```python
from build123d import *

# Parameters (mm, degrees)
SKETCH_1_W          = 20
SKETCH_1_H          = 20
SKETCH_1_W_2        = 17
SKETCH_1_H_2        = 17
EXTRUDE_1_DEPTH     = 415
SKETCH_5_R          = 1.6
CUT_EXTRUDE_4_DEPTH = 416.601973046


with BuildPart() as part:
    # 草图1 → 凸台-拉伸1 (new body)
    with BuildSketch(Plane.XY):
        Rectangle(SKETCH_1_W, SKETCH_1_H)
        Rectangle(SKETCH_1_W_2, SKETCH_1_H_2, mode=Mode.SUBTRACT)
    extrude(amount=EXTRUDE_1_DEPTH)

    # 草图5 → 切除-拉伸4 (cut, through all)
    with BuildSketch(Plane.XZ.offset(10)):
        with Locations(Location((0, 10, 0), (0, 0, 270))):
            Circle(SKETCH_5_R)
        with Locations(Location((0, 30, 0), (0, 0, 270))):
            Circle(SKETCH_5_R)
        with Locations(Location((0, 50, 0), (0, 0, 270))):
            Circle(SKETCH_5_R)
        with Locations(Location((0, 70, 0), (0, 0, 270))):
            Circle(SKETCH_5_R)
        with Locations(Location((0, 90, 0), (0, 0, 270))):
            Circle(SKETCH_5_R)
        with Locations(Location((0, 110, 0), (0, 0, 270))):
            Circle(SKETCH_5_R)
        with Locations(Location((0, 130, 0), (0, 0, 270))):
            Circle(SKETCH_5_R)
        with Locations(Location((0, 150, 0), (0, 0, 270))):
            Circle(SKETCH_5_R)
        with Locations(Location((0, 170, 0), (0, 0, 270))):
            Circle(SKETCH_5_R)
        with Locations(Location((0, 190, 0), (0, 0, 270))):
            Circle(SKETCH_5_R)
        with Locations(Location((0, 210, 0), (0, 0, 270))):
            Circle(SKETCH_5_R)
        with Locations(Location((0, 230, 0), (0, 0, 270))):
            Circle(SKETCH_5_R)
    extrude(amount=-CUT_EXTRUDE_4_DEPTH, mode=Mode.SUBTRACT)


solid = part.part
```
Can you work these out from the model? Positions are in its coordinate system, mm. A direction names the side the tool comes from. Round coordinates to 2 decimals unless told otherwise and drop trailing zeros. Loops run counter-clockwise (first coordinate to the right, second up) from the corner with the lowest first, then second, coordinate; pieces in that order, holes last. Notation, with made-up numbers: M 74.25,7 L 78.25,7 A23 ccw 78.25,17 Z; hole C 89.25,-13.75 d6. An arc over 180 degrees is marked long. Answer as a JSON object with one key per item and string values. Group by question number.
Q1. Please list where these lines run through material, in increasing order: L1, parallel to X at y = 2.75, z = 202; L2, parallel to X at y = 9.25, z = 210.
Q2. Imagine slicing it at A-A, the plane y = 5.5. Please give me the cut outline in (x, z).
Q3. Imagine slicing it at B-B, the plane z = 303.5. Please give me the cut outline in (x, y), then the cut area to 3 significant figures.
Q4. On a 3-axis mill with a long thin cutter (end or side, diameter ignored), from which of +Z, -Z, +X, -X, +Y, -Y can I reach the whole of each face in a straight line? I mean faces 1 (the flat face through (0, -10, 205)), 2 (the flat face through (8.5, 0, 205)). Say none if no direction works.
Q5. We'd pull the mould along X, two halves only. Please class faces 3 (the flat face through (0, 8.5, 205)), 4 (the flat face through (-10, 0, 205)), 5 (the flat face through (10, 0, 205)): +X half, -X half, draft (parallel to the pull), parting line (faces both ways), or undercut.
Findings:
{
 "1": {"L1": "x = -10 to -8.5, 8.5 to 10", "L2": "x = -10 to -1.6, 1.6 to 10"},
 "2": {"outline": "M -10,0 L -8.5,0 L -8.5,415 L -10,415 Z; M 8.5,0 L 10,0 L 10,415 L 8.5,415 Z"},
 "3": {"outline": "M -10,-10 L 10,-10 L 10,10 L -10,10 Z; hole M -8.5,-8.5 L 8.5,-8.5 L 8.5,8.5 L -8.5,8.5 Z", "area": "111 mm2"},
 "4": {"face 1": "+Z, -Z, +X, -X, -Y", "face 2": "+Z, -Z"},
 "5": {"face 3": "undercut", "face 4": "-X half", "face 5": "+X half"}
}
